Source: CAD feature listing. Evaluate the final solid. Frame: model axes, mm. A direction names the side the tool comes from. Round coordinates to 2 decimals unless told otherwise and drop trailing zeros. Order: outer loops, then holes, each group sorted by start corner. A loop starts at its lowest first (then second) coordinate and runs counter-clockwise, first axis right, second up. Notation, with made-up numbers: (82.5, 16) -> (100.5, 16) arc R27 cw to (100.5, 39) -> close; hole circle Ø1 at (-13.75, -18). An arc over 180 degrees is marked (long way). One line per item, written item: value. Start each with the question number.
1) Section D-D (x = 7.5). Return the cut outline in (y, z), and give its area (3 significant figures).
2) Section A-A (y = 0). Return the cut outline in (x, z), and give its area (3 significant figures).
3) Section B-B (x = 0). Return the cut outline in (y, z), and give its area (3 significant figures).
4) Ray query, L1, parallel to Y at x = 0, z = 13; L2, parallel to Y at x = 0, z = 3; L3, parallel to X at y = 2, z = -13. Return the intervals inside material, ascending.
5) Section C-C (y = 17.5). Return the cut outline in (x, z).
6) Mould query, pull axis Y, two halves, no side actions, for faces 6 (the face through (0, 5, -43)), 7 (the face through (-3, 1, 5)), 8 (the face through (-16, 16, 14)). Classes: pulls with the +Y half, pulls with the -Y half, needs draft (parallel to the pull), parting line crosses it, or undercut.
7) Reachability of faces 1 (the face through (-13, 0, -25)), 2 (the face through (0, -12.5, 11)), 3 (the face through (0, 0, -50)), 4 (the face through (0, -5, -43)), 5 (the face through (-23, 0, -30)) from +Z, -Z, +X, -X, +Y, -Y: full face, straight path, thin tool, end or side. Return the list, or none.
8) Pin query (flat end, axial travel): P1, Ø2.5, axis at x = 2, z = 8, coming from the +Y side; P2, Ø11, axis at y = 1.5, z = -21.5, coming from the -X side; P3, Ø3, axis at y = -16.5, z = 3.5, coming from the +X side. Return the tip coordinate at first contact, or that it passes through.
```python
from build123d import *

# Parameters (mm, degrees)
SKETCH_1_R      = 37.5
SKETCH_1_R_2    = 3
EXTRUDE_1_DEPTH = 5
EXTRUDE_START   = 10
SKETCH_2_R      = 37.5
EXTRUDE_2_DEPTH = 10
SKETCH_4_R      = 37.5
SKETCH_4_W      = 12
SKETCH_4_H      = 12
EXTRUDE_3_DEPTH = 5
SKETCH_6_R      = 37.5
SKETCH_6_W      = 12
SKETCH_6_H      = 25
EXTRUDE_4_DEPTH = 2
SKETCH_11_R     = 37.5
SKETCH_11_R_2   = 20
EXTRUDE_6_DEPTH = 2
SKETCH_13_W     = 10
SKETCH_13_H     = 10
EXTRUDE_7_DEPTH = 30
SKETCH_14_W     = 46
SKETCH_14_H     = 10
EXTRUDE_8_DEPTH = 10


with BuildPart() as part:
    # Эскиз1 → Бобышка-Вытянуть1 (new body)
    with BuildSketch(Plane.XY):
        Circle(SKETCH_1_R)
        Circle(SKETCH_1_R_2, mode=Mode.SUBTRACT)
    extrude(amount=EXTRUDE_1_DEPTH)

    # Эскиз2 → Бобышка-Вытянуть2 (add)
    with BuildSketch(Plane(origin=(0, 0, 0), x_dir=(-1, 0, 0), z_dir=(0, 0, -1)).offset(EXTRUDE_START)):
        Circle(SKETCH_2_R)
    extrude(amount=-EXTRUDE_2_DEPTH)

    # Эскиз4 → Бобышка-Вытянуть3 (add)
    with BuildSketch(Plane.XY.offset(5)):
        with Locations(Location((0, 0, 0), (0, 0, 180))):
            Circle(SKETCH_4_R)
        Rectangle(SKETCH_4_W, SKETCH_4_H, mode=Mode.SUBTRACT)
    extrude(amount=EXTRUDE_3_DEPTH)

    # Эскиз6 → Бобышка-Вытянуть4 (add)
    with BuildSketch(Plane.XY.offset(10)):
        with Locations(Location((0, 0, 0), (0, 0, 180))):
            Circle(SKETCH_6_R)
        Rectangle(SKETCH_6_W, SKETCH_6_H, mode=Mode.SUBTRACT)
    extrude(amount=EXTRUDE_4_DEPTH)

    # Эскиз11 → Бобышка-Вытянуть6 (add)
    with BuildSketch(Plane.XY.offset(12)):
        with Locations(Location((0, 0, 0), (0, 0, 180))):
            Circle(SKETCH_11_R)
        Circle(SKETCH_11_R_2, mode=Mode.SUBTRACT)
    extrude(amount=EXTRUDE_6_DEPTH)

    # Эскиз13 → Бобышка-Вытянуть7 (add)
    with BuildSketch(Plane(origin=(0, 0, -10), x_dir=(-1, 0, 0), z_dir=(0, 0, -1))):
        with Locations((-18, 0)):
            Rectangle(SKETCH_13_W, SKETCH_13_H)
        with Locations((18, 0)):
            Rectangle(SKETCH_13_W, SKETCH_13_H)
    extrude(amount=EXTRUDE_7_DEPTH)

    # Эскиз14 → Бобышка-Вытянуть8 (add)
    with BuildSketch(Plane(origin=(0, 0, -40), x_dir=(-1, 0, 0), z_dir=(0, 0, -1))):
        Rectangle(SKETCH_14_W, SKETCH_14_H)
    extrude(amount=EXTRUDE_8_DEPTH)


solid = part.part
```
Findings:
1. outline: (-36.74, -10) -> (36.74, -10) -> (36.74, 14) -> (18.54, 14) -> (18.54, 12) -> (-18.54, 12) -> (-18.54, 14) -> (-36.74, 14) -> close; (-5, -50) -> (5, -50) -> (5, -40) -> (-5, -40) -> close
1. area: 1,790 mm2
2. outline: (-37.5, -10) -> (-23, -10) -> (-23, -50) -> (23, -50) -> (23, -10) -> (37.5, -10) -> (37.5, 14) -> (20, 14) -> (20, 12) -> (6, 12) -> (6, 5) -> (3, 5) -> (3, 0) -> (-3, 0) -> (-3, 5) -> (-6, 5) -> (-6, 12) -> (-20, 12) -> (-20, 14) -> (-37.5, 14) -> close; hole (-13, -40) -> (13, -40) -> (13, -10) -> (-13, -10) -> close
2. area: 2,670 mm2
3. outline: (-37.5, -10) -> (37.5, -10) -> (37.5, 14) -> (20, 14) -> (20, 12) -> (12.5, 12) -> (12.5, 10) -> (6, 10) -> (6, 5) -> (3, 5) -> (3, 0) -> (-3, 0) -> (-3, 5) -> (-6, 5) -> (-6, 10) -> (-12.5, 10) -> (-12.5, 12) -> (-20, 12) -> (-20, 14) -> (-37.5, 14) -> close; (-5, -50) -> (5, -50) -> (5, -40) -> (-5, -40) -> close
3. area: 1,680 mm2
4. L1: -37.5 to -20, 20 to 37.5
4. L2: -37.5 to -3, 3 to 37.5
4. L3: -23 to -13, 13 to 23
5. outline: (-33.17, -10) -> (33.17, -10) -> (33.17, 14) -> (9.68, 14) -> (9.68, 12) -> (-9.68, 12) -> (-9.68, 14) -> (-33.17, 14) -> close
6. face 6: pulls with the +Y half
6. face 7: undercut
6. face 8: needs draft
7. face 1: +Y, -Y
7. face 2: +Z
7. face 3: -Z, +X, -X, +Y, -Y
7. face 4: -Z, +X, -X, -Y
7. face 5: -Z, -X, +Y, -Y
8. P1: y = 37.49
8. P2: x = -23
8. P3: x = 34.37
